Verification items for this drawing (mm, ordinates from the low corner). A direction names the side the tool comes from. Round coordinates to 2 decimals unless told otherwise and drop trailing zeros. Order: outer loops, then holes, each group sorted by start corner. A loop starts at its lowest first (then second) coordinate and runs counter-clockwise, first axis right, second up. Notation, with made-up numbers: M 30,85.5 L 41,85.5 A17 ccw 41,102.5 Z; hole C 35,49 d11. An arc over 180 degrees is marked long. One line per item, written item: value. Start each with the question number.
(1) Cross-section at A-A, the plane x = 21.5. Enter the section's corners in (y, z) (1 decimal).
(2) Depth check by flat-ended pin: pin 1 Ø1.5 at (x, y) = (18.5, 11.5) entering from -Z; pin 2 Ø1.5 at (x, z) = (21, 12.5) entering from -Y (3 decimals). Enter the tip coordinate at first touch or a pass-through.
(3) Release check for a two-part mould opening along Z. For the marked faces 1, 2 and 3 record: released by +Z, released by -Z, zero draft, split by the parting line, or undercut.
(4) Access from +Z, -Z, +X, -X, +Y, -Y to the whole of each face (thin tool, end or side, straight path). Record for the marked faces 4, 5 and 6.
(5) Thickness scan on L1, parallel to X at y = 6, z = 1.1; L2, parallel to Y at x = 30, z = 1.4; L3, parallel to Z at x = 10.5, y = 16.3 (1 decimal). Record the ranges inside material, lowest first.
(6) Cross-section at B-B, the plane z = 4. Enter the section's corners in (x, y) (3 decimals).
(7) Cross-section at C-C, the plane y = 3. Enter the section's corners in (x, z) (3 decimals).
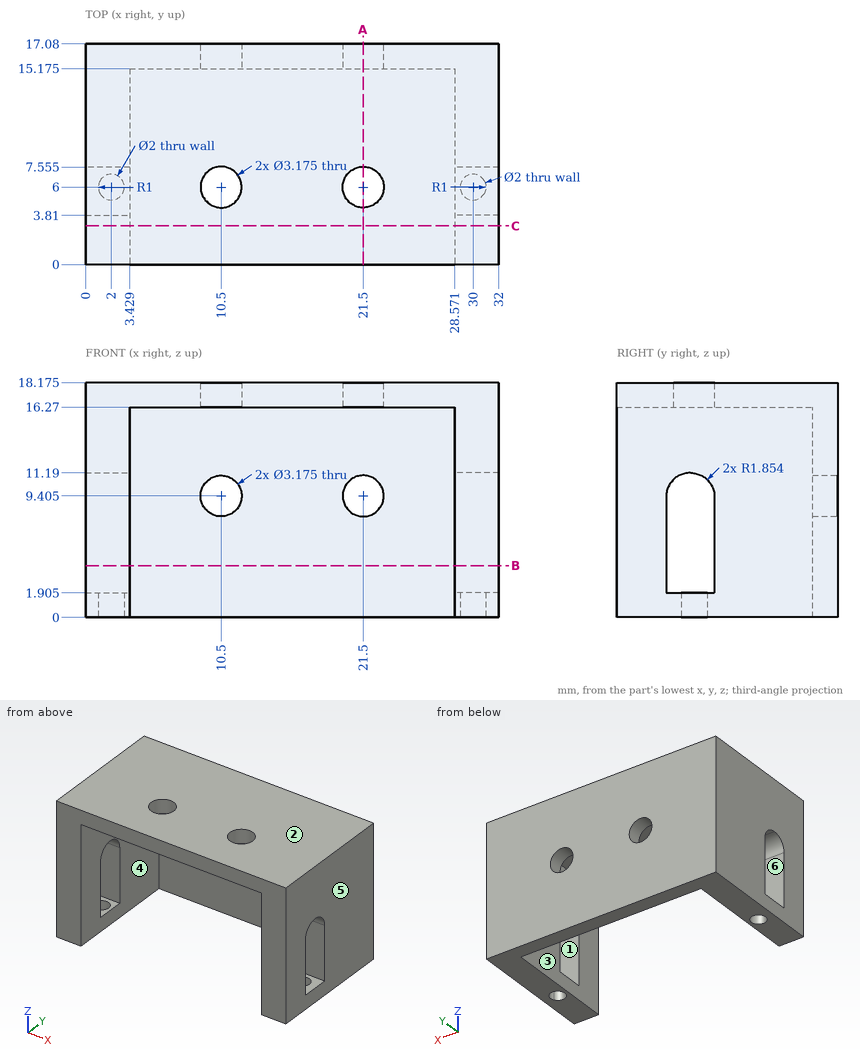
Values found:
1. outline: M 0,16.3 L 4.4,16.3 L 4.4,18.2 L 0,18.2 Z; M 7.6,16.3 L 15.2,16.3 L 15.2,11 L 17.1,11 L 17.1,18.2 L 7.6,18.2 Z; M 15.2,0 L 17.1,0 L 17.1,7.8 L 15.2,7.8 Z
2. pin 1: z = 16.27
2. pin 2: y = 15.175
3. face 1: undercut
3. face 2: released by +Z
3. face 3: zero draft
4. face 4: -Z, -Y
4. face 5: +Z, -Z, +X, +Y, -Y
4. face 6: +X, -X
5. L1: 0 to 1, 3 to 3.43, 28.57 to 29, 31 to 32
5. L2: 0 to 5, 7 to 17.08
5. L3: 0 to 7.8, 11 to 18.2
6. outline: M 0,0 L 3.429,0 L 3.429,3.81 L 0,3.81 Z; M 0,7.555 L 3.429,7.555 L 3.429,15.175 L 28.571,15.175 L 28.571,7.555 L 32,7.555 L 32,17.08 L 0,17.08 Z; M 28.571,0 L 32,0 L 32,3.81 L 28.571,3.81 Z
7. outline: M 0,0 L 3.429,0 L 3.429,16.27 L 28.571,16.27 L 28.571,0 L 32,0 L 32,18.175 L 0,18.175 Z
